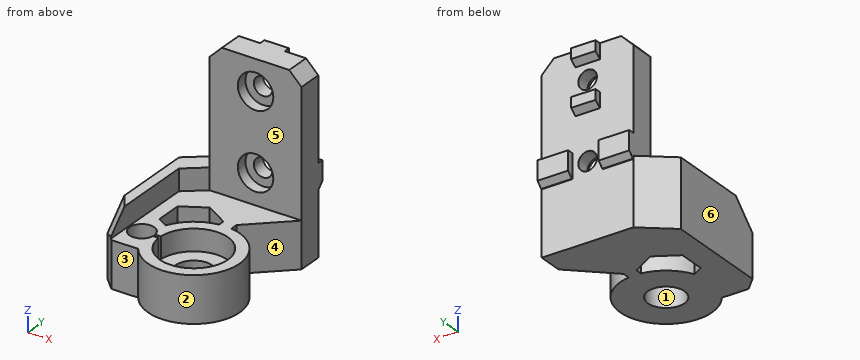
from build123d import *

# Parameters (mm, degrees)
F0_W           = 30
F0_H           = 60
F1_DEPTH       = 8
F2_D           = 6.1
F2_CBORE_D     = 11.6
F2_CBORE_DEPTH = 3.6
F3_R           = 6
F4_DEPTH       = 15
F6_DEPTH       = 12
F5_R           = 6
F7_DEPTH       = 7
F9_DEPTH       = 7
F10_SIZE       = 7
F11_W          = 8
F11_H          = 5
F11_W_2        = 10
F11_H_2        = 8
F12_DEPTH      = 2
F13_SIZE2      = 1.678189
F13_SIZE       = 1.99999
F13_2_SIZE2    = 1.678189
F13_2_SIZE     = 1.99999
F14_SIZE2      = 1.75
F14_SIZE       = 1.75
F15_T1_DEPTH   = 35.5734639037
F16_SIZE       = 3.49999
F17_SIZE       = 4


# Not quite as in the source:
# - a fillet or chamfer that OpenCascade refuses, or shapes differently, is made with other operations: its cross-section is extruded or revolved along the edge and cut away or added
# - a fillet or chamfer is up to 0.001 mm smaller than in the source, because OpenCascade refuses the exact size


with BuildPart() as f1:
    # F0 (on Front) → F1 (new body)
    with BuildSketch(Plane.XZ):
        with Locations((15, 30)):
            Rectangle(F0_W, F0_H)
    extrude(amount=-F1_DEPTH)

    # F2 (through all)
    with Locations(Plane.XZ):
        with Locations((15, 50), (15, 25)):
            CounterBoreHole(F2_D / 2, F2_CBORE_D / 2, F2_CBORE_DEPTH)

    # F3 (on face) → F4 (join)
    with BuildSketch(Plane(origin=(0, 0, 0), x_dir=(1, 0, 0), z_dir=(0, 0, -1))):
        with BuildLine():
            Line((-10, 0), (0, -8))
            Line((0, -8), (0, 0))
            Line((0, 0), (30, 0))
            Line((30, 0), (17, 12))
            Line((17, 12), (17, 14.4339312527))
            ThreePointArc((17, 14.4339312527), (27.843214237, 37.0493127477), (2.7807528874, 38))
            Line((2.7807528874, 38), (-10, 38))
            Line((-10, 38), (-10, 0))
        make_face()
        Polygon((-2, 12.3301270189), (-2, 20.9903810568), (1.4069435951, 22.9573808585), (5.5, 25.3205080757), (13, 20.9903810568), (13, 14.4339312527), (13, 12.3301270189), (5.5, 8), align=None, mode=Mode.SUBTRACT)
        with Locations((15, 29.3)):
            Circle(F3_R, mode=Mode.SUBTRACT)
        with BuildLine():
            Line((5.5, 25.3205080757), (1.4069435951, 22.9573808585))
            ThreePointArc((1.4069435951, 22.9573808585), (6.1147228345, 17.2148086613), (13, 14.4339312527))
            Line((13, 14.4339312527), (13, 20.9903810568))
            Line((13, 20.9903810568), (5.5, 25.3205080757))
        make_face()
    extrude(amount=-F4_DEPTH)

    # F5 (on face) → F6 (cut)
    with BuildSketch(Plane.XY.offset(15)):
        with BuildLine():
            ThreePointArc((2.0190172928, -29.8), (2.0422469022, -29.5504795042), (2.05, -29.3))
            ThreePointArc((2.05, -29.3), (2.0422469022, -29.0495204958), (2.0190172928, -28.8))
            ThreePointArc((2.0190172928, -28.8), (-6.05, -29.3), (2.0190172928, -29.8))
        make_face()
    extrude(amount=-F6_DEPTH, mode=Mode.SUBTRACT)

    # F5 (on face) → F7 (cut)
    with BuildSketch(Plane.XY.offset(15)):
        with BuildLine():
            ThreePointArc((2.0190172928, -28.8), (2.0422469022, -29.0495204958), (2.05, -29.3))
            ThreePointArc((2.05, -29.3), (2.0422469022, -29.5504795042), (2.0190172928, -29.8))
            Line((2.0190172928, -29.8), (3.8612164039, -29.8))
            ThreePointArc((3.8612164039, -29.8), (3.85, -29.3), (3.8612164039, -28.8))
            Line((3.8612164039, -28.8), (2.0190172928, -28.8))
        make_face()
        with BuildLine():
            ThreePointArc((26.15, -29.3), (15.2500628959, -18.1528044537), (3.8612164039, -28.8))
            ThreePointArc((3.8612164039, -28.8), (3.85, -29.3), (3.8612164039, -29.8))
            ThreePointArc((3.8612164039, -29.8), (15.2500628959, -40.4471955463), (26.15, -29.3))
        make_face()
        with Locations((15, -29.3)):
            Circle(F5_R, mode=Mode.SUBTRACT)
        with Locations((15, -29.3)):
            Circle(F5_R)
    extrude(amount=-F7_DEPTH, mode=Mode.SUBTRACT)

    # F8 (on face) → F9 (join)
    with BuildSketch(Plane.XY.offset(15)):
        Polygon((-6.5, -5.2), (0, 0), (0, 8), (-10, 0), (-10, -38), (-6.5, -38), align=None)
    extrude(amount=F9_DEPTH)

    # F10
    f10_edges = [f1.edges().sort_by_distance(p)[0] for p in [
        (-8.25, -38, 22),
    ]]
    chamfer(f10_edges, length=F10_SIZE)

    # F11 (on face) → F12 (join)
    with BuildSketch(Plane(origin=(0, 8, 0), x_dir=(-1, 0, 0), z_dir=(0, 1, 0))):
        with Locations((-15, 57.5)):
            Rectangle(F11_W, F11_H)
        with Locations((-15, 42.5)):
            Rectangle(F11_W, F11_H)
        Polygon((0, 22), (0, 29), (-10, 29), (-10, 21), (0, 21), align=None)
        with Locations((-25, 25)):
            Rectangle(F11_W_2, F11_H_2)
    extrude(amount=F12_DEPTH)

    # F13 (size 2 and 1.6781992624 in the source; OpenCascade refuses exactly that, so slightly less here)
    f13_edges = [f1.edges().sort_by_distance(p)[0] for p in [
        (15, 10, 55),
    ]]
    f13_side = f1.faces().sort_by_distance((15, 9, 55))[0]
    chamfer(f13_edges, length=F13_SIZE, length2=F13_SIZE2, reference=f13_side)

    # F13#2 (size 2 and 1.6781992624 in the source; OpenCascade refuses exactly that, so slightly less here)
    f13_2_edges = [f1.edges().sort_by_distance(p)[0] for p in [
        (15, 10, 40),
    ]]
    f13_2_side = f1.faces().sort_by_distance((15, 9, 40))[0]
    chamfer(f13_2_edges, length=F13_2_SIZE, length2=F13_2_SIZE2, reference=f13_2_side)

    # F14
    f14_edges = [f1.edges().sort_by_distance(p)[0] for p in [
        (25, 10, 21),
        (5, 10, 21),
    ]]
    chamfer(f14_edges, length=F14_SIZE, length2=F14_SIZE2)

    # F15: chamfer of 4 on 1 edges, made by hand

    # F15_s2 → F15_t1 (cut)
    with BuildSketch(Plane.XY.offset(-10.2867319519)):
        Polygon((-6, -38), (-10, -34), (-10, -38), align=None)
    extrude(amount=F15_T1_DEPTH, mode=Mode.SUBTRACT)

    # F16 (size 3.5 in the source; OpenCascade refuses exactly that, so slightly less here)
    f16_edges = [f1.edges().sort_by_distance(p)[0] for p in [
        (-10, -32.5, 20.5),
    ]]
    chamfer(f16_edges, length=F16_SIZE)

    # F17
    f17_edges = [f1.edges().sort_by_distance(p)[0] for p in [
        (30, 4, 60),
        (0, 4, 60),
    ]]
    chamfer(f17_edges, length=F17_SIZE)


solid = f1.part
The model under review builds one solid part; all positions refer to its coordinate system, in mm. Face numbers are marked on the shaded views. A direction names the side the tool comes from. Round coordinates to 2 decimals unless told otherwise and drop trailing zeros. Order: outer loops, then holes, each group sorted by start corner. A loop starts at its lowest first (then second) coordinate and runs counter-clockwise, first axis right, second up. Notation, with made-up numbers: (-40, -33) - (-25, -33) arc R14 cw to (-25, -18) - close; hole circle Ø10 at (15.25, 18.5). An arc over 180 degrees is marked (long way). Use one line per item in the form item = value.
Q1. Tool access review of the marked faces 4, 5 and 6: name each direction out of +Z, -Z, +X, -X, +Y, -Y from which nothing blocks a thin tool from reaching the whole face with its end or side.
Response values:
face_4 = +Z, -Z, +X
face_5 = +Z, +X, -Y
face_6 = +Z, -Z, -X, +Y, -Y
Q2. Mouldability with a two-part tool opening along X and no side actions: class the marked faces 1, 2 and 3 as pulls with the +X half, pulls with the -X half, needs draft (parallel to the pull), parting line crosses it, or undercut.
Response values:
face_1 = undercut
face_2 = parting line crosses it
face_3 = needs draft
Q3. Add section A-A on z = 25. Give the boundary of the cut face in (x, y), then the cut area to 3 significant figures.
Response values:
outline = (0, 0) - (9.2, 0) - (9.2, 3.6) - (11.95, 3.6) - (11.95, 8) - (10, 8) - (10, 10) - (0, 10) - close; (18.05, 3.6) - (20.8, 3.6) - (20.8, 0) - (30, 0) - (30, 10) - (20, 10) - (20, 8) - (18.05, 8) - close
area = 211 mm^2
Q4. Clearance check with flat-ended pins moving along their axes: P1, Ø10, axis at x = 0, z = 13.5, coming from the -Y side; P2, Ø1.2, axis at y = -12.5, z = 4, coming from the +X side; P3, Ø4, axis at y = -16, z = 23.5, coming from the +X side; P4, Ø5.5, axis at x = 15, z = 50, coming from the +Y side. State where each tip first meets the part, or that it passes through.
Response values:
P1 = -40.48
P2 = 17.11
P3 = -6.5
P4 = through
Q5. Add section B-B on x = 25. Give the boundary of the cut face in (y, z).
Response values:
outline = (-40.48, 0) - (-18.12, 0) - (-18.12, 15) - (-24.37, 15) - (-24.37, 8) - (-34.23, 8) - (-34.23, 15) - (-40.48, 15) - close; (-4.62, 0) - (8, 0) - (8, 21) - (8.25, 21) - (10, 22.75) - (10, 29) - (8, 29) - (8, 60) - (0, 60) - (0, 15) - (-4.62, 15) - close
Q6. Add section C-C on y = -27. Give the boundary of the cut face in (x, z), then the cut area to 3 significant figures.
Response values:
outline = (-10, 0) - (9.46, 0) - (9.46, 8) - (4.09, 8) - (4.09, 15) - (1.33, 15) - (1.33, 3) - (-5.33, 3) - (-5.33, 15) - (-6.5, 15) - (-6.5, 22) - (-9.33, 22) - (-10, 21.05) - close; (20.54, 0) - (29.82, 0) - (29.82, 15) - (25.91, 15) - (25.91, 8) - (20.54, 8) - close
area = 300 mm^2
Q7. To check wall thickness, follow line 1 (X direction, y = -29, z = 6); line 2 (Z direction, x = 15, y = 6); line 3 (Z direction, x = 15, y = 1.7). State the ranges of each line that lie inside material, in increasing order.
Response values:
line_1 = -10 to -6.04, 2.04 to 9.01, 20.99 to 30
line_2 = 0 to 21.95, 28.05 to 46.95, 53.05 to 60
line_3 = 0 to 19.2, 30.8 to 44.2, 55.8 to 60
Q8. Add section D-D on z = 50. Give the boundary of the cut face in (x, y), then the cut area to 3 significant figures.
Response values:
outline = (0, 0) - (9.2, 0) - (9.2, 3.6) - (11.95, 3.6) - (11.95, 8) - (0, 8) - close; (18.05, 3.6) - (20.8, 3.6) - (20.8, 0) - (30, 0) - (30, 8) - (18.05, 8) - close
area = 171 mm^2
